The model under review builds one solid part; all positions refer to its coordinate system, in mm. A direction names the side the tool comes from. Coordinates: 2 decimals unless noted, no trailing zeros. Loops run counter-clockwise (first coordinate to the right, second up) from the corner with the lowest first, then second, coordinate; pieces in that order, holes last. Notation, with made-up numbers: M 80,43.25 L 133,43.25 A22 ccw 133,51.25 Z; hole C 58,-25 d10. An arc over 180 degrees is marked long. Return JSON: item names as keys, results as strings.
```python
from build123d import *

# Parameters (mm, degrees)
SKETCH1_R           = 3.075
BOSS_EXTRUDE1_DEPTH = 2
BOSS_EXTRUDE2_DEPTH = 7


with BuildPart() as part:
    # Sketch1 → Boss-Extrude1 (new body)
    with BuildSketch(Plane(origin=(0, 0, 0), x_dir=(1, 0, 0), z_dir=(0, 1, 0))):
        Polygon((69.882295615, -141.15690287), (82.382295615, -133.65690287), (90.871460172, -120.65690287), (69.882295615, -120.65690287), align=None)
        with Locations(Location((76.382295615, -129.15690287, 0), (0, 0, 270))):
            Circle(SKETCH1_R, mode=Mode.SUBTRACT)
    extrude(amount=BOSS_EXTRUDE1_DEPTH)

    # Sketch2 → Boss-Extrude2 (add)
    with BuildSketch(Plane(origin=(0, 0, 0), x_dir=(-1, 0, 0), z_dir=(0, -1, 0))):
        Polygon((-69.882295615, -141.15690287), (-82.382295615, -133.65690287), (-90.871460172, -120.65690287), (-81.03443504, -132.776732853), (-71.882295615, -138.268016507), (-69.882295615, -139.65690287), align=None)
    extrude(amount=-BOSS_EXTRUDE2_DEPTH)


solid = part.part
```
1. Insertion check: pin 1 Ø12 at (x, z) = (78.5, 125.5) entering from +Y; pin 2 Ø1.5 at (y, z) = (4, 137) entering from +X; pin 3 Ø3 at (y, z) = (5.5, 125) entering from -X. Each pin has a flat end and moves straight along its axis. Give the tip position at first contact, or say it passes through.
Check values:
{"pin 1": "y = 2", "pin 2": "x = 78.06", "pin 3": "x = 86.13"}
2. Add section B-B on z = 130. Give the boundary of the cut face in (x, y), plus the area to 3 significant figures.
Check values:
{"outline": "M 69.88,0 L 73.43,0 L 73.43,2 L 69.88,2 Z; M 79.34,0 L 84.77,0 L 84.77,7 L 83.29,7 L 83.29,2 L 79.34,2 Z", "area": "25.4 mm²"}
3. Machinability: for faces 4 (the face through (80, 7, 134)), 5 (the face through (76.522, 4.465, 135.484)), which of the approach directions +Z, -Z, +X, -X, +Y, -Y give a long, thin tool a straight path to every point of the face, cutting with its end or side? Answer none if there is none.
Check values:
{"face 4": "+Z, -Z, +X, -X, +Y", "face 5": "-Z, -X, +Y"}
4. Add section A-A on x = 75.5. Give the boundary of the cut face in (y, z), plus the area to 3 significant figures.
Check values:
{"outline": "M 0,120.66 L 2,120.66 L 2,126.21 L 0,126.21 Z; M 0,132.1 L 2,132.1 L 2,136.1 L 7,136.1 L 7,137.79 L 0,137.79 Z", "area": "30.9 mm²"}
5. Add section D-D on z = 134.5. Give the boundary of the cut face in (x, y).
Check values:
{"outline": "M 69.88,0 L 80.98,0 L 80.98,7 L 78.16,7 L 78.16,2 L 69.88,2 Z"}
6. The part is to be moulded in two halves that separate along X. For faces 1 (the face through (73.38, 0.99, 128.49)), 2 (the face through (86.022, 4.465, 126.632)), 3 (the face through (76.04, 3.45, 137.46)), say which applies: released by +X, released by -X, zero draft, split by the parting line, or undercut.
Check values:
{"face 1": "undercut", "face 2": "released by -X", "face 3": "released by +X"}
7. To check wall thickness, follow line 1 (Y direction, x = 75.5, z = 124.25); line 2 (X direction, y = 1.75, z = 130); line 3 (Z direction, x = 79, y = 4). State the ranges of each line that lie inside material, in increasing order.
Check values:
{"line 1": "0 to 2", "line 2": "69.88 to 73.43, 79.34 to 84.77", "line 3": "134 to 135.69"}
8. Add section C-C on y = 6.75. Give the boundary of the cut face in (x, z).
Check values:
{"outline": "M 69.88,139.66 L 71.88,138.27 L 81.03,132.78 L 90.87,120.66 L 82.38,133.66 L 69.88,141.16 Z"}
